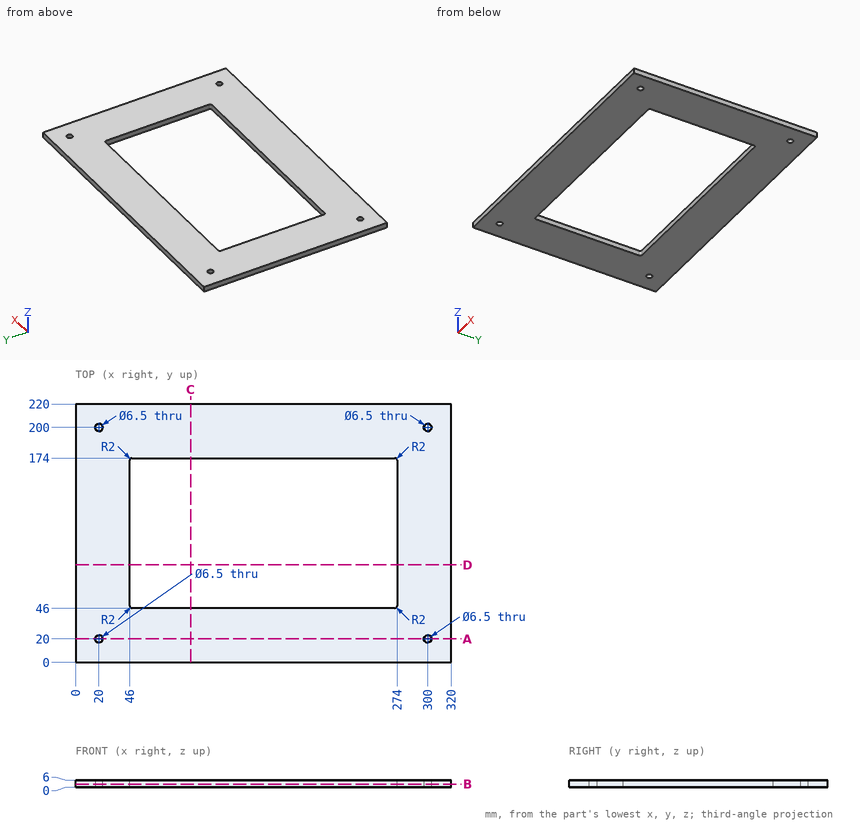
Geometry check sheet. Reference: drawing and pictorial views, mm from the part's lowest x, y, z. Round coordinates to 2 decimals unless told otherwise and drop trailing zeros. Order: outer loops, then holes, each group sorted by start corner. A loop starts at its lowest first (then second) coordinate and runs counter-clockwise, first axis right, second up. Notation, with made-up numbers: (-21.75, 14.5) - (13.25, 14.5) arc R25 ccw to (13.25, 34.5) - close; hole circle Ø1 at (-15.5, -9.5). An arc over 180 degrees is marked (long way). Use a Markdown table: item, result. Add a question column.
1) Thickness scan on line 1 along X through (y, z) = (20, 3.7); line 2 along Y through (x, z) = (300, 2.1); line 3 along Y through (x, z) = (129, 4.75). Record the ranges inside material, lowest first.
2) Section check B-B (z = 2.65). Record the cut outline in (x, y).
3) Section check D-D (y = 83). Record the cut outline in (x, z), then the cut area to 3 significant figures.
4) Section check C-C (x = 98). Record the cut outline in (y, z).
5) Section check A-A (y = 20). Record the cut outline in (x, z).
Established:
| question | item | result |
|---|---|---|
| 1 | line 1 | 0 to 16.75, 23.25 to 296.75, 303.25 to 320 |
| 1 | line 2 | 0 to 16.75, 23.25 to 196.75, 203.25 to 220 |
| 1 | line 3 | 0 to 46, 174 to 220 |
| 2 | outline | (0, 0) - (320, 0) - (320, 220) - (0, 220) - close; hole circle Ø6.5 at (20, 20); hole circle Ø6.5 at (20, 200); hole (46, 48) arc R2 ccw to (48, 46) - (272, 46) arc R2 ccw to (274, 48) - (274, 172) arc R2 ccw to (272, 174) - (48, 174) arc R2 ccw to (46, 172) - close; hole circle Ø6.5 at (300, 20); hole circle Ø6.5 at (300, 200) |
| 3 | outline | (0, 0) - (46, 0) - (46, 6) - (0, 6) - close; (274, 0) - (320, 0) - (320, 6) - (274, 6) - close |
| 3 | area | 552 mm2 |
| 4 | outline | (0, 0) - (46, 0) - (46, 6) - (0, 6) - close; (174, 0) - (220, 0) - (220, 6) - (174, 6) - close |
| 5 | outline | (0, 0) - (16.75, 0) - (16.75, 6) - (0, 6) - close; (23.25, 0) - (296.75, 0) - (296.75, 6) - (23.25, 6) - close; (303.25, 0) - (320, 0) - (320, 6) - (303.25, 6) - close |
